from build123d import *

# Parameters (mm, degrees)
F2_SIZE = 0.8
F3_SIZE = 0.4


with BuildPart() as f1:
    # F0 (on Right) → F1 (revolve)
    with BuildSketch(Plane.YZ):
        Polygon((-2, 4), (-2, 0), (0.8, 0), (0.8, 3), (0, 3), (0, 4), align=None)
    revolve(axis=Axis((0, -0.6, 0), (0, -1, 0)))

    # F2
    f2_edges = [f1.edges().sort_by_distance(p)[0] for p in [
        (0, -2, -4),
    ]]
    chamfer(f2_edges, length=F2_SIZE)

    # F3
    f3_edges = [f1.edges().sort_by_distance(p)[0] for p in [
        (0, 0.8, -3),
    ]]
    chamfer(f3_edges, length=F3_SIZE)


solid = f1.part
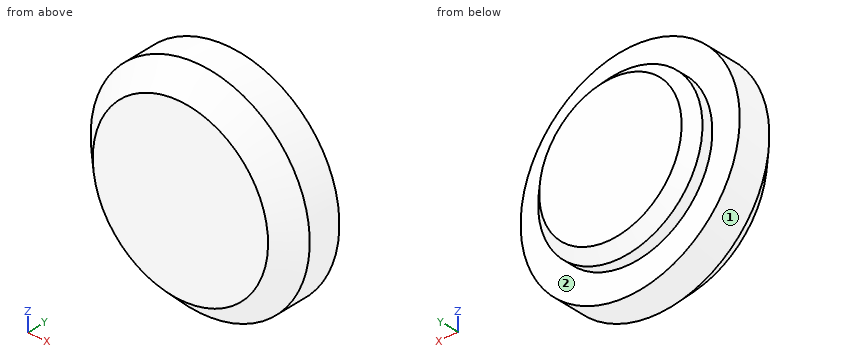
The listing builds one solid part. Answer for the finished solid, in the listing's coordinates (mm). Face numbers are marked on the shaded views. A direction names the side the tool comes from. Coordinates: 2 decimals unless noted, no trailing zeros. Order: outer loops, then holes, each group sorted by start corner. A loop starts at its lowest first (then second) coordinate and runs counter-clockwise, first axis right, second up.
Q1. A cutting plane is placed at B-B, the plane z = 0. Write down the section's boundary in (x, y), and give its area (3 significant figures).
Q2. Which of the six approach directions +Z, -Z, +X, -X, +Y, -Y give full straight-line access (tool end or side, diameter ignored) to the marked faces 1 and 2?
Q3. A cutting plane is placed at C-C, the plane y = -0.7. Write down the section's boundary in (x, z), and give its area (3 significant figures).
Q4. Consider line 1 (Y direction, x = 3, z = -1); line 2 (Z direction, x = 3.5, y = -0.35); line 3 (X direction, y = -1.05, z = -2.25). Determine where each line is inside the solid, lowest interval first.
Q5. Given P1, Ø1.5, axis at x = -2, y = 0, coming from the +Z side; P2, Ø1.5, axis at x = -1, y = -1, coming from the +Z side, each flat-ended and moving along its own axis, determine where each tip first touches the part or whether it passes through.
Q6. A cutting plane is placed at D-D, the plane y = -1.8. Write down the section's boundary in (x, z), and give its area (3 significant figures).
Q7. A cutting plane is placed at A-A, the plane x = 0. Write down the section's boundary in (y, z), and give its area (3 significant figures).
Answers follow:
1. outline: (-4, -1.2) - (-3.2, -2) - (3.2, -2) - (4, -1.2) - (4, 0) - (3, 0) - (3, 0.4) - (2.6, 0.8) - (-2.6, 0.8) - (-3, 0.4) - (-3, 0) - (-4, 0) - close
1. area: 20.0 mm2
2. face 1: +Y, -Y
2. face 2: +Y
3. outline: circle Ø8 at (0, 0)
3. area: 50.3 mm2
4. line 1: y = -2 to 0
4. line 2: z = -1.94 to 1.94
4. line 3: x = -3.31 to 3.31
5. P1: stops at z = 3.8
5. P2: stops at z = 3.99
6. outline: circle Ø6.8 at (0, 0)
6. area: 36.3 mm2
7. outline: (-2, -3.2) - (-1.2, -4) - (0, -4) - (0, -3) - (0.4, -3) - (0.8, -2.6) - (0.8, 2.6) - (0.4, 3) - (0, 3) - (0, 4) - (-1.2, 4) - (-2, 3.2) - close
7. area: 20.0 mm2
